Input: part model. Units: mm. Frame: model coordinates. A direction names the side the tool comes from. Give positions to 0.01 mm unless a question says otherwise; leave off trailing zeros. Write each loop counter-clockwise with the first axis right and the second up, starting at its lowest first coordinate (ties: lowest second). Pieces come first, ordered by that corner, then holes. Notation, with made-up numbers: (79, -27) - (111, -27) arc R18 cw to (111, 0) - close; hole circle Ø7 at (76.25, 86.25). An arc over 180 degrees is marked (long way). Use a Markdown table: item, result. Add a question column.
1. Section query C-C, the plane z = 15. Count the separate pieces of the cut face and the enclosed holes in it, plus the area to 3 significant figures.
2. Set-up query: faces 1 (the cylindrical face through (-3.34, -12.38, 8.54)), 2 (the flat face through (-34, -10, 4.5)), 3 (the flat face through (33, -10, 4.5)), 4 (the flat face through (18.76, 27.99, 12.48)). Return all of +Z, -Z, +X, -X, +Y, -Y with unobstructed straight access to the full face (end or side cutting, diameter ignored); none if empty.
3. Section query A-A, the plane x = 0. Return loops of the section in (y, z), plus the area to 3 significant figures.
4. Mould query, pull axis Y, two halves, no side actions, for faces 5 (the flat face through (-10, 34, 4.5)), 6 (the cylindrical face through (12.38, -3.34, 8.54)), 7 (the flat face through (-15.09, -30.64, 12.48)). Classes: released by +Y, released by -Y, zero draft, split by the parting line, or undercut.
5. Material intervals for probe 1 along Y at (x, z) = (24.5, 16.25); probe 2 along X at (y, z) = (-37.5, 20); probe 3 along X at (y, z) = (39.5, 15), sorted ascending.
6. Section query B-B, the plane y = 0. Return loops of the section in (x, z).
7. Pin query (flat end, axial travel): pin 1 (3 mm diameter, centred on x = 27.5, z = 5.5, fed in from +Y); pin 2 (10.5 mm diameter, centred on x = -28, z = 20, fed in from -Y); pin 3 (2 mm diameter, centred on x = 6, y = -23, fed in from -Z); pin 4 (23 mm diameter, centred on x = 0, y = 0, fed in from +Z). Return the tip coordinate at first contact, or that it passes through.
```python
from build123d import *

# Parameters (mm, degrees)
SKETCH1_R           = 46.6725
BOSS_EXTRUDE1_DEPTH = 4.5
BOSS_EXTRUDE2_START = -4.5
BOSS_EXTRUDE2_DEPTH = 25.4


with BuildPart() as part:
    # Sketch1 → Boss-Extrude1 (new body)
    with BuildSketch(Plane.XY):
        Circle(SKETCH1_R)
        with BuildLine():
            Line((-2.927883194, 8.3225), (2.927883194, 8.3225))
            ThreePointArc((2.927883194, 8.3225), (0, -8.8225), (-2.927883194, 8.3225))
        make_face(mode=Mode.SUBTRACT)
    extrude(amount=BOSS_EXTRUDE1_DEPTH)

    # Sketch2 → Boss-Extrude2 (add)
    with BuildSketch(Plane.XY.offset(4.5).offset(BOSS_EXTRUDE2_START)):
        with BuildLine():
            Line((-2.25, 46.618234161), (-2.25, 13.778350254))
            ThreePointArc((-2.25, 13.778350254), (-3.318707206, 12.385583908), (-4.940617969, 13.057401343))
            Line((-4.940617969, 13.057401343), (-21.360559922, 41.497575063))
            ThreePointArc((-21.360559922, 41.497575063), (-23.33625, 40.419570658), (-25.257674239, 39.247575063))
            Line((-25.257674239, 39.247575063), (-8.837732286, 10.807401343))
            ThreePointArc((-8.837732286, 10.807401343), (-9.066876702, 9.066876702), (-10.807401343, 8.837732286))
            Line((-10.807401343, 8.837732286), (-39.247575063, 25.257674239))
            ThreePointArc((-39.247575063, 25.257674239), (-40.419570658, 23.33625), (-41.497575063, 21.360559922))
            Line((-41.497575063, 21.360559922), (-13.057401343, 4.940617969))
            ThreePointArc((-13.057401343, 4.940617969), (-12.385583908, 3.318707206), (-13.778350254, 2.25))
            Line((-13.778350254, 2.25), (-46.618234161, 2.25))
            ThreePointArc((-46.618234161, 2.25), (-46.6725, 0), (-46.618234161, -2.25))
            Line((-46.618234161, -2.25), (-13.778350254, -2.25))
            ThreePointArc((-13.778350254, -2.25), (-12.385583908, -3.318707206), (-13.057401343, -4.940617969))
            Line((-13.057401343, -4.940617969), (-41.497575063, -21.360559922))
            ThreePointArc((-41.497575063, -21.360559922), (-40.419570658, -23.33625), (-39.247575063, -25.257674239))
            Line((-39.247575063, -25.257674239), (-10.807401343, -8.837732286))
            ThreePointArc((-10.807401343, -8.837732286), (-9.066876702, -9.066876702), (-8.837732286, -10.807401343))
            Line((-8.837732286, -10.807401343), (-25.257674239, -39.247575063))
            ThreePointArc((-25.257674239, -39.247575063), (-23.33625, -40.419570658), (-21.360559922, -41.497575063))
            Line((-21.360559922, -41.497575063), (-4.940617969, -13.057401343))
            ThreePointArc((-4.940617969, -13.057401343), (-3.318707206, -12.385583908), (-2.25, -13.778350254))
            Line((-2.25, -13.778350254), (-2.25, -46.618234161))
            ThreePointArc((-2.25, -46.618234161), (0, -46.6725), (2.25, -46.618234161))
            Line((2.25, -46.618234161), (2.25, -13.778350254))
            ThreePointArc((2.25, -13.778350254), (3.318707206, -12.385583908), (4.940617969, -13.057401343))
            Line((4.940617969, -13.057401343), (21.360559922, -41.497575063))
            ThreePointArc((21.360559922, -41.497575063), (23.33625, -40.419570658), (25.257674239, -39.247575063))
            Line((25.257674239, -39.247575063), (8.837732286, -10.807401343))
            ThreePointArc((8.837732286, -10.807401343), (9.066876702, -9.066876702), (10.807401343, -8.837732286))
            Line((10.807401343, -8.837732286), (39.247575063, -25.257674239))
            ThreePointArc((39.247575063, -25.257674239), (40.419570658, -23.33625), (41.497575063, -21.360559922))
            Line((41.497575063, -21.360559922), (13.057401343, -4.940617969))
            ThreePointArc((13.057401343, -4.940617969), (12.385583908, -3.318707206), (13.778350254, -2.25))
            Line((13.778350254, -2.25), (46.618234161, -2.25))
            ThreePointArc((46.618234161, -2.25), (46.6725, 0), (46.618234161, 2.25))
            Line((46.618234161, 2.25), (13.778350254, 2.25))
            ThreePointArc((13.778350254, 2.25), (12.385583908, 3.318707206), (13.057401343, 4.940617969))
            Line((13.057401343, 4.940617969), (41.497575063, 21.360559922))
            ThreePointArc((41.497575063, 21.360559922), (40.419570658, 23.33625), (39.247575063, 25.257674239))
            Line((39.247575063, 25.257674239), (10.807401343, 8.837732286))
            ThreePointArc((10.807401343, 8.837732286), (9.066876702, 9.066876702), (8.837732286, 10.807401343))
            Line((8.837732286, 10.807401343), (25.257674239, 39.247575063))
            ThreePointArc((25.257674239, 39.247575063), (23.33625, 40.419570658), (21.360559922, 41.497575063))
            Line((21.360559922, 41.497575063), (4.940617969, 13.057401343))
            ThreePointArc((4.940617969, 13.057401343), (3.318707206, 12.385583908), (2.25, 13.778350254))
            Line((2.25, 13.778350254), (2.25, 46.618234161))
            ThreePointArc((2.25, 46.618234161), (0, 46.6725), (-2.25, 46.618234161))
        make_face()
        with BuildLine():
            Line((2.927883194, 8.3225), (-2.927883194, 8.3225))
            ThreePointArc((-2.927883194, 8.3225), (0, -8.8225), (2.927883194, 8.3225))
        make_face(mode=Mode.SUBTRACT)
    extrude(amount=BOSS_EXTRUDE2_DEPTH)

    # Sketch3 → Cut-Revolve1 (revolve, cut)
    with BuildSketch(Plane(origin=(0, 0, 0), x_dir=(1, 0, 0), z_dir=(0, 1, 0)), mode=Mode.PRIVATE) as cut_revolve1_sk:
        Polygon((-24.13, -12.7), (-6.35, -12.7), (-6.35, -25.4), (-35.56, -25.4), align=None)
    revolve(cut_revolve1_sk.sketch.rotate(Axis((0, 0, 0), (0, 0, 1)), 2.76320082), axis=Axis((0, 0, 0), (0, 0, 1)), mode=Mode.SUBTRACT)


solid = part.part
```
Result sheet:
| question | item | result |
|---|---|---|
| 1 | separate pieces | 12 |
| 1 | enclosed holes | 0 |
| 1 | area | 1,110 mm² |
| 2 | face 1 | +Z, -Y |
| 2 | face 2 | +Z, -X |
| 2 | face 3 | +Z, +X |
| 2 | face 4 | +Z |
| 3 | outline | (-46.67, 0) - (-8.82, 0) - (-8.82, 12.7) - (-24.13, 12.7) - (-35.56, 25.4) - (-46.67, 25.4) - close; (8.32, 0) - (46.67, 0) - (46.67, 25.4) - (35.56, 25.4) - (24.13, 12.7) - (8.32, 12.7) - close |
| 3 | area | 1,400 mm² |
| 4 | face 5 | zero draft |
| 4 | face 6 | undercut |
| 4 | face 7 | released by -Y |
| 5 | probe 1 | y = -39.72 to -37.94, -16.74 to -12.1, 12.1 to 16.74, 37.94 to 39.72 |
| 5 | probe 2 | x = -24.25 to -19.05, -2.25 to 2.25, 19.05 to 24.25 |
| 5 | probe 3 | x = -24.86 to -20.21, -2.25 to 2.25, 20.21 to 24.86 |
| 6 | outline | (-46.67, 0) - (-8.82, 0) - (-8.82, 12.7) - (-24.13, 12.7) - (-35.56, 25.4) - (-46.67, 25.4) - close; (8.82, 0) - (46.67, 0) - (46.67, 25.4) - (35.56, 25.4) - (24.13, 12.7) - (8.82, 12.7) - close |
| 7 | pin 1 | stops at y = 38.5 |
| 7 | pin 2 | stops at y = -40.75 |
| 7 | pin 3 | stops at z = 0 |
| 7 | pin 4 | stops at z = 12.7 |
